Autodesk Inventor part; units mm, degrees
ref_plane "Work Plane1" through (3.048, -55.7199, -88.0008) normal (1, 0, 0) x (0, 0.7407, 0.6718)
ref_plane "Work Plane3" through (-20.1841, -15.6194, -46.4564) normal (0, 0, 1) x (0.8084, 0.5887, 0)
ref_plane "YZ Plane" through (0, 0, 0) normal (1, 0, 0) x (0, 1, 0)
sketch "Sketch1" plane through (0, 0, 0) normal (1, 0, 0) x (0, 1, 0)
  line L0 (-24.1055, -88.5873) -> (-15.6118, -88.5873) construction
  line L1 (-20.9777, -35.0252) -> (-12.3846, 2.8126) construction
  line L2 (-11.1876, -82.4913) -> (-20.9871, -36.3884) construction
  line L3 (-10.1392, 12.7) -> (5.4091, 12.7)
  line L4 (5.4091, 12.7) -> (14.913, 2.8103)
  line L5 (14.913, 2.8103) -> (-0.1161, -33.4438)
  line L6 (-0.1161, -33.4438) -> (-0.1161, -88.5873)
  line L7 (-0.1161, -88.5873) -> (-9.8919, -88.5873)
  line L8 (-9.8919, -88.5873) -> (-21.1322, -35.7057)
  line L9 (-21.1322, -35.7057) -> (-10.1392, 12.7)
  line L10 (-0.1161, -27.3073) -> (-0.1161, -82.4913) construction
  arc A0 (9.8983, -7.957) -> (-12.3846, 2.8126) centre (0, 0) ccw construction
  point P0 (0, 0)
ref_plane "Work Plane1" through (3.048, -55.7199, -88.0008) normal (1, 0, 0) x (0, 0.7407, 0.6718)
extrude "Extrusion1" add sketch "Sketch1" along normal up to surface (3.048 mm away)
ref_plane "Work Plane2" through (86.0885, -0.1204, -88.5873) normal (0, 0, -1) x (0, -1, 0)
sketch "Sketch3" plane through (86.0885, -0.1204, -88.5873) normal (0, 0, -1) x (0, -1, 0)
  circle A0 centre (12.6956, 103.4693) radius 9.525
  line L0 (12.6956, 89.0216) -> (0.1835, 96.2455)
  line L1 (0.1835, 96.2455) -> (0.1835, 110.6932)
  line L2 (0.1835, 110.6932) -> (12.6956, 117.9171)
  line L3 (12.6956, 117.9171) -> (25.2077, 110.6932)
  line L4 (25.2077, 110.6932) -> (25.2077, 96.2455)
  line L5 (25.2077, 96.2455) -> (12.6956, 89.0216)
  point P0 (-0.1204, 86.0885)
ref_plane "Work Plane3" through (-20.1841, -15.6194, -46.4564) normal (0, 0, 1) x (0.8084, 0.5887, 0)
extrude "Extrusion2" add sketch "Sketch3" against normal up to surface (42.131 mm away) contours A0 | L0 L1 L2 L3 L4 L5
sketch "Sketch4" plane through (0, 0, 0) normal (-1, 0, 0) x (0, 0, 1)
  line L0 (-88.5873, -9.8919) -> (-88.5873, -0.1161)
  line L1 (-88.5873, -0.1161) -> (-33.4438, -0.1161)
  line L2 (-88.5873, -0.304) -> (-46.4564, -0.304)
  line L3 (-84.2988, -0.304) -> (-84.0662, -10.8529)
  line L4 (-35.7057, -21.1322) -> (-88.5873, -9.8919)
  point P0 (0, 0)
extrude "Extrusion3" add sketch "Sketch4" along normal blind 12.7
sketch "Sketch5" plane through (3.048, -0.1161, -88.5873) normal (0, 0, -1) x (-1, 0, 0)
  point P0 (3.048, 0.1161)
properties part number "ArmSolenoidBoundingBoc"
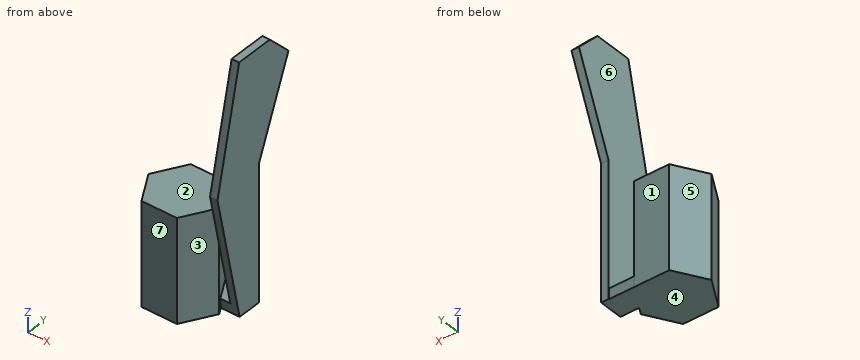
Here's how the part is built. I have some questions about the finished solid (model axes, mm). Face numbers are marked on the shaded views. A direction names the side the tool comes from. Round coordinates to 2 decimals unless told otherwise and drop trailing zeros. Order: outer loops, then holes, each group sorted by start corner. A loop starts at its lowest first (then second) coordinate and runs counter-clockwise, first axis right, second up. Notation, with made-up numbers: M -16,-25 L 12,-25 A20 cw 12,5 Z; hole C -3.5,4 d10. An arc over 180 degrees is marked long. Return JSON: item names as keys, results as strings. Group by question number.
1. If we section it at C-C on x = -9: List the corners of the cut face in (y, z) for me, then the cut area to 3 significant figures.
2. If we section it at A-A on z = -70.5: List the corners of the cut face in (x, y) for me.
3. Please list where these lines run through material, in increasing order: probe 1 along Z at (x, y) = (-15, -7); probe 2 along X at (y, z) = (2, -10.5); probe 3 along X at (y, z) = (-2, -64).
4. If we section it at B-B on y = -18: List the corners of the cut face in (x, z) for me, then the cut area to 3 significant figures.
5. I'm going to push flat-ended pins straight in: pin 1 Ø2.5 at (x, z) = (1.5, -71) entering from +Y; pin 2 Ø3.5 at (x, z) = (-2.5, -86) entering from +Y; pin 3 Ø12.5 at (x, y) = (-24.5, -8.5) entering from +Z; pin 4 Ø8 at (x, y) = (-15, 4.5) entering from -Z (3 decimals). Where does each tip first touch, or does it pass through?
6. If we mould it in two halves opening along X, with no side actions, what happens to the marked faces 5, 6 and 7? For each: pulls with the +X half, pulls with the -X half, needs draft (parallel to the pull), parting line crosses it, or undercut.
7. On a 3-axis mill with a long thin cutter (end or side, diameter ignored), from which of +Z, -Z, +X, -X, +Y, -Y can I reach the whole of each face in a straight line? I mean the marked faces 1, 2, 3 and 4. Say none if no direction works.
8. If we section it at D-D on z = -52: List the corners of the cut face in (x, y) for me.
Reply:
{
 "1": {"outline": "M -23.32,-88.59 L -0.3,-88.59 L -0.3,-84.3 L -2.31,-84.25 L -2.31,-46.46 L -23.32,-46.46 Z", "area": "894 mm^2"},
 "2": {"outline": "M -31.83,-12.82 L -24.6,-25.33 L -10.16,-25.33 L -2.93,-12.82 L -10.16,-0.3 L -24.6,-0.3 Z; M 0,-13.74 L 3.05,-13.74 L 3.05,-0.12 L 0,-0.12 Z"},
 "3": {"probe 1": "-88.59 to -46.46", "probe 2": "0 to 3.05", "probe 3": "-25.58 to -9.18, 0 to 3.05"},
 "4": {"outline": "M -28.84,-88.59 L -5.93,-88.59 L -5.93,-46.46 L -28.84,-46.46 Z; M 0,-50.44 L 3.05,-50.44 L 3.05,-21.91 L 0,-21.91 Z", "area": "1,050 mm^2"},
 "5": {"pin 1": "y = -0.12", "pin 2": "y = -0.3", "pin 3": "z = -46.46", "pin 4": "through"},
 "6": {"face 5": "pulls with the -X half", "face 6": "undercut", "face 7": "needs draft"},
 "7": {"face 1": "+Z, -Z, -X, +Y", "face 2": "+Z, -X, +Y, -Y", "face 3": "+Z, -Z, -Y", "face 4": "-Z, +X, -X, +Y, -Y"},
 "8": {"outline": "M -31.83,-12.82 L -24.6,-25.33 L -10.16,-25.33 L -2.93,-12.82 L -10.16,-0.3 L -24.6,-0.3 Z; M 0,-17.67 L 3.05,-17.67 L 3.05,-0.12 L 0,-0.12 Z"}
}
